```python
from build123d import *

# Parameters (mm, degrees)
SKETCH_1_R          = 1.5
EXTRUDE_1_DEPTH     = 2
SKETCH_2_R          = 2.95
EXTRUDE_2_DEPTH     = 0.95
CUT_EXTRUDE_1_DEPTH = 0.6
SKETCH_1_8_R        = 1.5
EXTRUDE_5_DEPTH     = 5


with BuildPart() as part:
    # Sketch 1 → Extrude 1 (new body)
    with BuildSketch(Plane(origin=(0, 0, 0), x_dir=(1, 0, 0), z_dir=(0, 1, 0))):
        with Locations(Location((0, 0, 0), (0, 0, 270))):
            Circle(SKETCH_1_R)
    extrude(amount=EXTRUDE_1_DEPTH)

    # Sketch 2 → Extrude 2 (add)
    with BuildSketch(Plane(origin=(0, 0, 0), x_dir=(-1, 0, 0), z_dir=(0, 1, 0))):
        with Locations(Location((0, 0, 0), (0, 0, 90))):
            Circle(SKETCH_2_R)
    extrude(amount=-EXTRUDE_2_DEPTH)

    # Sketch 4 → Cut-Revolve 1 (revolve, cut)
    with BuildSketch(Plane(origin=(0, 0, 0), x_dir=(0, 0, -1), z_dir=(1, 0, 0))):
        with BuildLine():
            Line((-2.901374674, 0), (-2.95, 0))
            Line((-2.95, 0), (-2.95, -0.95))
            Line((-2.95, -0.95), (-2.901374674, -0.95))
            ThreePointArc((-2.901374674, -0.95), (-2.94, -0.475), (-2.901374674, 0))
        make_face()
    revolve(axis=Axis((0, 3.165730861, 0), (0, -1, 0)), mode=Mode.SUBTRACT)

    # Sketch 3 → Cut-Extrude 1 (cut)
    with BuildSketch(Plane.XZ.offset(0.95)):
        Polygon((1.5, -0.4), (1.5, 0.4), (0.4, 0.4), (0.4, 1.5), (-0.4, 1.5), (-0.4, 0.4), (-1.5, 0.4), (-1.5, -0.4), (-0.4, -0.4), (-0.4, -1.5), (0.4, -1.5), (0.4, -0.4), align=None)
    extrude(amount=-CUT_EXTRUDE_1_DEPTH, mode=Mode.SUBTRACT)

    # Sketch 1_8 → Extrude 5 (add)
    with BuildSketch(Plane(origin=(0, 0, 0), x_dir=(1, 0, 0), z_dir=(0, 1, 0))):
        with Locations(Location((0, 0, 0), (0, 0, 270))):
            Circle(SKETCH_1_8_R)
    extrude(amount=EXTRUDE_5_DEPTH)


solid = part.part
```
Read the model definition and answer for the solid it produces. Units are mm, in the model's axes. A direction names the side the tool comes from. Give positions to 0.01 mm unless a question says otherwise; leave off trailing zeros. Loops run counter-clockwise (first coordinate to the right, second up) from the corner with the lowest first, then second, coordinate; pieces in that order, holes last.
Item 1: Find the intervals of material crossed by line 1 along Y through (x, z) = (0.8, -1.8); line 2 along X through (y, z) = (3.95, -0.35); line 3 along Z through (x, y) = (-1.95, -0.4), in increasing order.
Item 2: For faces 1 (the flat face through (-1, -0.95, 1)), 2 (the flat face through (-1.2, 0, 1.2)), determine the directions among +Z, -Z, +X, -X, +Y, -Y from which every point of the face is accessible in a straight line to the end or side of a thin tool.
Item 3: Each of these flat-tipped pins is pushed along its axis until it touches: pin 1 Ø3 at (y, z) = (0.5, 2) entering from +X; pin 2 Ø0.5 at (x, y) = (1, -0.5) entering from +Z; pin 3 Ø0.7 at (x, y) = (-0.5, -1) entering from -Z; pin 4 Ø3.5 at (x, z) = (0.5, 0) entering from -Y. Where does it stop, or does it pass through?
Item 4: The part is cut by section B-B (x = -0.2). Write down the section's boundary in (y, z) (3 decimals), and give its area (3 significant figures).
Item 5: The part is cut by section D-D (x = -2.1). Write down the section's boundary in (y, z) (3 decimals).
Item 6: The part is cut by section C-C (y = 3.55). Write down the section's boundary in (x, z), and give its area (3 significant figures).
Item 7: The part is cut by section A-A (z = 0). Write down the section's boundary in (x, y) (3 decimals), and give its area (3 significant figures).
Item 8: The mould has two halves that part along Z. Classify faces 3 (the cylindrical face through (0.45, 2.46, 1.43)), 4 (the flat face through (0, 5, 0)), 5 (the flat face through (0, -0.35, 0)): released by +Z, released by -Z, zero draft, split by the parting line, or undercut.
Taken from the geometry:
1. line 1: y = -0.95 to 0
1. line 2: x = -1.46 to 1.46
1. line 3: z = -2.2 to 2.2
2. face 1: +Z, -Z, +X, -X, -Y
2. face 2: +Y
3. pin 1: stops at x = 2.85
3. pin 2: stops at z = 2.84
3. pin 3: stops at z = -2.92
3. pin 4: stops at y = -0.95
4. outline: (-0.95, -2.894) arc R2.933 ccw to (0, -2.894) - (0, -1.487) - (5, -1.487) - (5, 1.487) - (0, 1.487) - (0, 2.894) arc R2.933 ccw to (-0.95, 2.894) - (-0.95, 1.5) - (-0.35, 1.5) - (-0.35, -1.5) - (-0.95, -1.5) - close
4. area: 18.6 mm2
5. outline: (-0.95, -2.002) arc R2.058 ccw to (0, -2.002) - (0, 2.002) arc R2.058 ccw to (-0.95, 2.002) - close
6. outline: circle Ø3 at (0, 0)
6. area: 7.07 mm2
7. outline: (-2.901, -0.95) - (-1.5, -0.95) - (-1.5, -0.35) - (1.5, -0.35) - (1.5, -0.95) - (2.901, -0.95) arc R2.94 ccw to (2.901, 0) - (1.5, 0) - (1.5, 5) - (-1.5, 5) - (-1.5, 0) - (-2.901, 0) arc R2.94 ccw to start
7. area: 18.8 mm2
8. face 3: split by the parting line
8. face 4: zero draft
8. face 5: undercut
